```python
from build123d import *

# Parameters (mm, degrees)
F1_DEPTH = 25.4
F2_R     = 10.329538
F3_DEPTH = 25.401
F4_R     = 10.647707
F5_DEPTH = 25.4
F7_DEPTH = 25.4
F9_DEPTH = 25.4


with BuildPart() as f1:
    # F0 (on Front) → F1 (new body)
    with BuildSketch(Plane.XZ):
        Polygon((-67.925481, 0.01739), (-33.977801, -58.816497), (33.94768, -58.833887), (67.925481, -0.01739), (33.977801, 58.816497), (-33.94768, 58.833887), align=None)
    extrude(amount=F1_DEPTH)

    # F2 (on face) → F3 (cut, through all)
    with BuildSketch(Plane.XZ.offset(25.4)):
        with Locations((-23.201194, 29.740747)):
            Circle(F2_R)
    extrude(amount=-F3_DEPTH, mode=Mode.SUBTRACT)

    # F4 (on Front) → F5 (cut)
    with BuildSketch(Plane.XZ):
        with Locations((23.428654, 30.081941)):
            Circle(F4_R)
    extrude(amount=F5_DEPTH, mode=Mode.SUBTRACT)

    # F6 (on face) → F7 (cut)
    with BuildSketch(Plane.XZ.offset(25.4)):
        Polygon((7.633303, -4.40709), (0, 8.814179), (-7.633303, -4.40709), align=None)
    extrude(amount=-F7_DEPTH, mode=Mode.SUBTRACT)

    # F8 (on face) → F9 (cut)
    with BuildSketch(Plane.XZ.offset(25.4)):
        with BuildLine():
            Line((-18.615896, -23.2519), (-33.279214, -23.2519))
            ThreePointArc((-33.279214, -23.2519), (0, -40.5975), (33.279214, -23.2519))
            Line((33.279214, -23.2519), (19.561792, -22.46194))
            ThreePointArc((19.561792, -22.46194), (0.616189, -29.779569), (-18.615896, -23.2519))
        make_face()
    extrude(amount=-F9_DEPTH, mode=Mode.SUBTRACT)


solid = f1.part
```
CAD build for the part. Positions are in the model's coordinates, mm. A direction names the side the tool comes from. Round coordinates to 2 decimals unless told otherwise and drop trailing zeros. Loops run counter-clockwise (first coordinate to the right, second up) from the corner with the lowest first, then second, coordinate; pieces in that order, holes last. Notation, with made-up numbers: M 22,25 L 51,25 A23 ccw 51,50 Z; hole C 78,-11 d8. An arc over 180 degrees is marked long. Use a Markdown table: item, result. Add a question column.
(1) Drill centre lines: line 1 (Z direction, x = 22.5, y = -22); line 2 (Z direction, x = -2.5, y = -13.5); line 3 (X direction, y = -16.25, z = 3.5). Where is each one in solid material? Low to high.
(2) Cut at B-B (z = 2). Give the cut face in (x, y).
(3) Flat gauge pins, fed straight in: pin 1 (4 mm diameter, centred on x = -23.5, y = -3, fed in from -Z); pin 2 (12 mm diameter, centred on y = -10, z = 22, fed in from +X); pin 3 (10 mm diameter, centred on y = -8, z = 6, fed in from +X). Where does each tip first touch, or does it go through?
(4) Cut at D-D (z = -28). Give the cut face in (x, y), and give its area (3 significant figures).
(5) Cut at C-C (y = -6.5). Give the cut face in (x, z) (1 decimal), and give its area (3 significant figures).
(6) Pull direction X, two halves, no side cores. Call faces 3 (the face through (14, -25.4, 1)), 4 (the face through (-50.699, -12.522, 29.837)), 5 (the face through (28.342, -12.522, 20.636)): +X half, -X half, draft (parallel to the pull), parting line (faces both ways), or undercut.
(7) Cut at A-A (x = -3.5). Give the cut face in (y, z), and give its area (3 significant figures).
(8) Which spindle directions (+Z, -Z, +X, -X, +Y, -Y) get a long thin tool onto all of the face, cutting with end or side? Do faces 1 (the face through (-26, -13, -23.252)), 2 (the face through (14, 0, 1)). Say none if no direction does.
Geometry says:
| question | item | result |
|---|---|---|
| 1 | line 1 | z = -58.83 to -33.79, -22.63 to 19.47, 40.69 to 58.82 |
| 1 | line 2 | z = -58.82 to -40.52, -29.68 to -4.41, 4.48 to 58.83 |
| 1 | line 3 | x = -65.91 to -3.07, 3.07 to 65.9 |
| 2 | outline | M -66.78,-25.4 L -3.93,-25.4 L -3.93,0 L -66.78,0 Z; M 3.93,-25.4 L 66.76,-25.4 L 66.76,0 L 3.93,0 Z |
| 3 | pin 1 | stops at z = -58.82 |
| 3 | pin 2 | stops at x = 58.68 |
| 3 | pin 3 | stops at x = 67.34 |
| 4 | outline | M -51.76,-25.4 L -29.4,-25.4 L -29.4,0 L -51.76,0 Z; M -10.16,-25.4 L 10.16,-25.4 L 10.16,0 L -10.16,0 Z; M 29.4,-25.4 L 51.76,-25.4 L 51.76,0 L 29.4,0 Z |
| 4 | area | 1,650 mm² |
| 5 | outline | M -67.9,0 L -34,-58.8 L 33.9,-58.8 L 67.9,0 L 34,58.8 L -33.9,58.8 Z; hole C -23.2,29.7 d20.7; hole M -33.3,-23.3 A40.6 ccw 33.3,-23.3 L 19.6,-22.5 A29.8 cw -18.6,-23.3 Z; hole M -7.6,-4.4 L 7.6,-4.4 L 0,8.8 Z; hole C 23.4,30.1 d21.3 |
| 5 | area | 10,500 mm² |
| 6 | face 3 | draft |
| 6 | face 4 | -X half |
| 6 | face 5 | undercut |
| 7 | outline | M -25.4,-58.82 L 0,-58.82 L 0,-40.45 L -25.4,-40.45 Z; M -25.4,-29.58 L 0,-29.58 L 0,-4.41 L -25.4,-4.41 Z; M -25.4,2.75 L 0,2.75 L 0,58.83 L -25.4,58.83 Z |
| 7 | area | 2,530 mm² |
| 8 | face 1 | +Y, -Y |
| 8 | face 2 | +Z, -Z, +X, -X, +Y |
